Here's the drawing with two shaded views (mm, measured from the low corner). I have some questions. Round coordinates to 2 decimals unless told otherwise and drop trailing zeros. Order: outer loops, then holes, each group sorted by start corner. A loop starts at its lowest first (then second) coordinate and runs counter-clockwise, first axis right, second up.
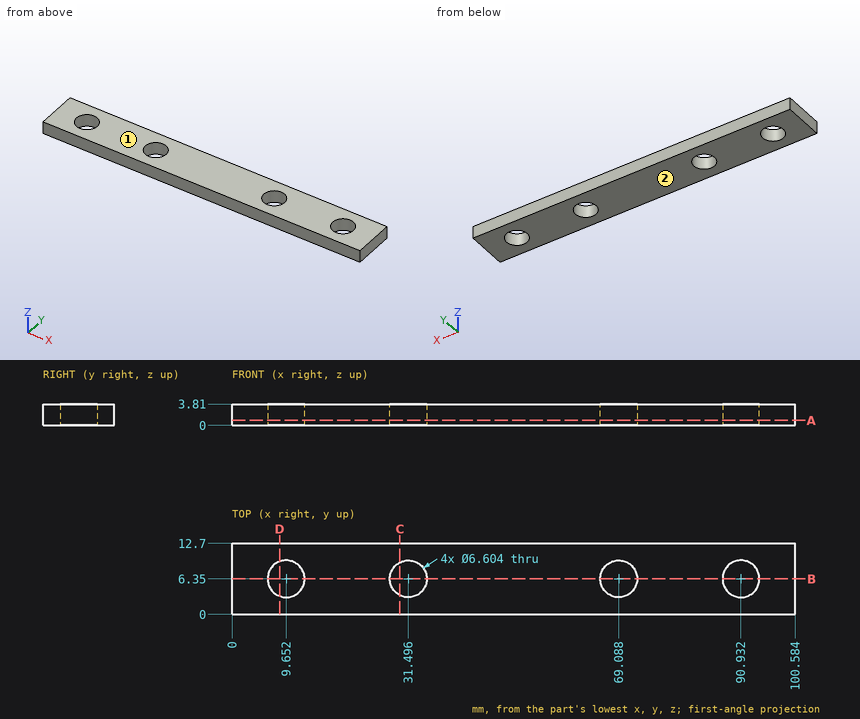
1. If we section it at B-B, the plane y = 6.35: Write out the boundary of the cut face in (x, z).
Evaluation:
outline: (0, 0) - (6.35, 0) - (6.35, 3.81) - (0, 3.81) - close; (12.95, 0) - (28.19, 0) - (28.19, 3.81) - (12.95, 3.81) - close; (34.8, 0) - (65.79, 0) - (65.79, 3.81) - (34.8, 3.81) - close; (72.39, 0) - (87.63, 0) - (87.63, 3.81) - (72.39, 3.81) - close; (94.23, 0) - (100.58, 0) - (100.58, 3.81) - (94.23, 3.81) - close
2. If we section it at A-A, the plane z = 0.9: Write out the boundary of the cut face in (x, y).
Evaluation:
outline: (0, 0) - (100.58, 0) - (100.58, 12.7) - (0, 12.7) - close; hole circle Ø6.6 at (9.65, 6.35); hole circle Ø6.6 at (31.5, 6.35); hole circle Ø6.6 at (69.09, 6.35); hole circle Ø6.6 at (90.93, 6.35)
3. If we section it at D-D, the plane x = 8.5: Write out the boundary of the cut face in (y, z), and give its area (3 significant figures).
Evaluation:
outline: (0, 0) - (3.26, 0) - (3.26, 3.81) - (0, 3.81) - close; (9.44, 0) - (12.7, 0) - (12.7, 3.81) - (9.44, 3.81) - close
area: 24.8 mm2
4. I need wall thicknesses on probe 1 along X at (y, z) = (8.25, 1.15); probe 2 along X at (y, z) = (4, 3.35). Which ranges of each line are inside material? Lowest first, please.
Evaluation:
probe 1: x = 0 to 6.95, 12.35 to 28.8, 34.2 to 66.39, 71.79 to 88.23, 93.63 to 100.58
probe 2: x = 0 to 7.33, 11.97 to 29.18, 33.82 to 66.77, 71.41 to 88.61, 93.25 to 100.58
5. If we section it at C-C, the plane x = 30: Write out the boundary of the cut face in (y, z).
Evaluation:
outline: (0, 0) - (3.41, 0) - (3.41, 3.81) - (0, 3.81) - close; (9.29, 0) - (12.7, 0) - (12.7, 3.81) - (9.29, 3.81) - close
6. If we mould it in two halves opening along Z, with no side actions, what happens to the marked faces 1 and 2? For each: released by +Z, released by -Z, zero draft, split by the parting line, or undercut.
Evaluation:
face 1: released by +Z
face 2: released by -Z
